Here's how the part is built. I have some questions about the finished solid (model axes, mm). Face numbers are marked on the shaded views. A direction names the side the tool comes from. Give positions to 0.01 mm unless a question says otherwise; leave off trailing zeros. Loops run counter-clockwise (first coordinate to the right, second up) from the corner with the lowest first, then second, coordinate; pieces in that order, holes last. Notation, with made-up numbers: (55.5, -20) - (86.5, -20) arc R26 cw to (86.5, 15) - close; hole circle Ø1 at (27.5, 54). An arc over 180 degrees is marked (long way). Use a Markdown table: item, result.
from build123d import *

# Parameters (mm, degrees)
F2_R     = 6.35
F3_DEPTH = 10.161
F4_COUNT = 6


with BuildPart() as f1:
    # F0 (on Right) → F1 (revolve)
    with BuildSketch(Plane.YZ):
        Polygon((-63.5, 0), (-12.7, 0), (-12.7, 5.08), (-25.4, 5.08), (-25.4, 7.62), (-27.94, 7.62), (-27.94, 10.16), (-60.96, 10.16), (-60.96, 7.62), (-63.5, 7.62), align=None)
    revolve(axis=Axis((0, 0, 21.0262340249), (0, 0, 1)))

    # F2 (on face) → F3 (cut, through all)
    with BuildSketch(Plane.XY.offset(10.16)):
        with Locations((0, -44.45)):
            Circle(F2_R)
    f3 = extrude(amount=-F3_DEPTH, mode=Mode.SUBTRACT)

    # F4: F3 ×6 about axis
    f4_axis = Axis((0, 0, 10.16), (0, 0, 1))
    for i in range(1, F4_COUNT):
        add(f3.rotate(f4_axis, i * 360 / F4_COUNT), mode=Mode.SUBTRACT)


solid = f1.part
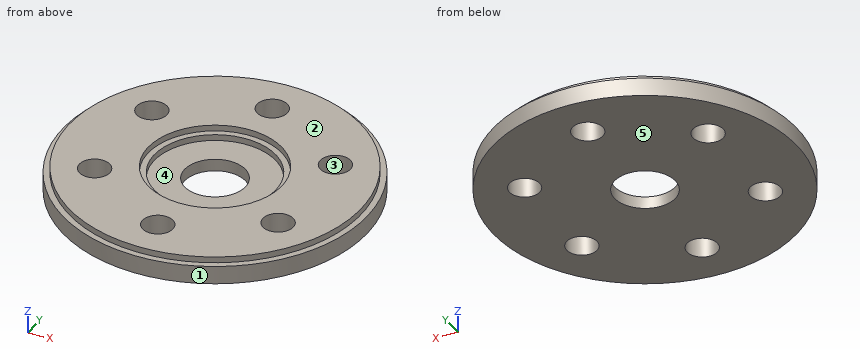
(1) If I drill on line 1 (X direction, y = 0, z = 7.1); line 2 (X direction, y = 0, z = 8.35); line 3 (X direction, y = -27, z = 1.5), over which ranges is the centre line in solid material (lowest first)?
A:
| item | result |
|---|---|
| line 1 | -63.5 to -25.4, 25.4 to 63.5 |
| line 2 | -60.96 to -27.94, 27.94 to 60.96 |
| line 3 | -57.47 to -42.68, -34.31 to 34.31, 42.68 to 57.47 |
(2) Suppose I cut it at A-A on y = 0. Write out the boundary of the cut face in (x, z), plus the area to 3 significant figures.
A:
| item | result |
|---|---|
| outline | (-63.5, 0) - (-12.7, 0) - (-12.7, 5.08) - (-25.4, 5.08) - (-25.4, 7.62) - (-27.94, 7.62) - (-27.94, 10.16) - (-60.96, 10.16) - (-60.96, 7.62) - (-63.5, 7.62) - close; (12.7, 0) - (63.5, 0) - (63.5, 7.62) - (60.96, 7.62) - (60.96, 10.16) - (27.94, 10.16) - (27.94, 7.62) - (25.4, 7.62) - (25.4, 5.08) - (12.7, 5.08) - close |
| area | 877 mm2 |
(3) Suppose I cut it at B-B on x = -3.5. Write out the boundary of the cut face in (y, z).
A:
| item | result |
|---|---|
| outline | (-63.4, 0) - (-49.75, 0) - (-49.75, 10.16) - (-60.86, 10.16) - (-60.86, 7.62) - (-63.4, 7.62) - close; (-39.15, 0) - (-12.21, 0) - (-12.21, 5.08) - (-25.16, 5.08) - (-25.16, 7.62) - (-27.72, 7.62) - (-27.72, 10.16) - (-39.15, 10.16) - close; (12.21, 0) - (39.15, 0) - (39.15, 10.16) - (27.72, 10.16) - (27.72, 7.62) - (25.16, 7.62) - (25.16, 5.08) - (12.21, 5.08) - close; (49.75, 0) - (63.4, 0) - (63.4, 7.62) - (60.86, 7.62) - (60.86, 10.16) - (49.75, 10.16) - close |
(4) Suppose I cut it at D-D on y = -44.45. Write out the boundary of the cut face in (x, z), plus the area to 3 significant figures.
A:
| item | result |
|---|---|
| outline | (-45.35, 0) - (-6.35, 0) - (-6.35, 10.16) - (-41.72, 10.16) - (-41.72, 7.62) - (-45.35, 7.62) - close; (6.35, 0) - (45.35, 0) - (45.35, 7.62) - (41.72, 7.62) - (41.72, 10.16) - (6.35, 10.16) - close |
| area | 774 mm2 |
(5) Will these pins go through, and if not, where does the flat tip stop? pin 1 (5 mm diameter, centred on x = -25.5, z = 5, fed in from -Y); pin 2 (3 mm diameter, centred on y = -28, z = 8, fed in from +X); pin 3 (3 mm diameter, centred on x = 5, z = 4.5, fed in from -Y).
A:
| item | result |
|---|---|
| pin 1 | y = -59.19 |
| pin 2 | x = 57.68 |
| pin 3 | y = -63.4 |
(6) Suppose I cut it at C-C on x = 38. Write out the boundary of the cut face in (y, z).
A:
| item | result |
|---|---|
| outline | (-50.87, 0) - (-28.56, 0) - (-28.56, 10.16) - (-47.67, 10.16) - (-47.67, 7.62) - (-50.87, 7.62) - close; (-15.89, 0) - (15.89, 0) - (15.89, 10.16) - (-15.89, 10.16) - close; (28.56, 0) - (50.87, 0) - (50.87, 7.62) - (47.67, 7.62) - (47.67, 10.16) - (28.56, 10.16) - close |
(7) We'd pull the mould along Y, two halves only. Please class the marked faces 1, 2 and 3: pulls with the +Y half, pulls with the -Y half, needs draft (parallel to the pull), parting line crosses it, or undercut.
A:
| item | result |
|---|---|
| face 1 | parting line crosses it |
| face 2 | needs draft |
| face 3 | undercut |
(8) On a 3-axis mill with a long thin cutter (end or side, diameter ignored), from which of +Z, -Z, +X, -X, +Y, -Y can I reach the whole of each face in a straight line? I mean the marked faces 4 and 5. Say none if no direction works.
A:
| item | result |
|---|---|
| face 4 | +Z |
| face 5 | -Z, +X, -X, +Y, -Y |
